from build123d import *

# Parameters (mm, degrees)
SKETCH1_W                   = 6.35
SKETCH1_H                   = 158.75
BOSS_EXTRUDE1_DEPTH         = 31.75
SKETCH2_R                   = 3.048
AXLE_HOLES_DEPTH            = 7.35
F_3_0MM_DOWEL_HOLE2_D       = 3
SKETCH4_W                   = 6.0325
SKETCH4_H                   = 6.638636364
CHEESING_CUT_DEPTH          = 5.334
FILLET1_R                   = 2.54
F_3_0MM_DOWEL_HOLE1_D       = 3
M3X0_5_TAPPED_HOLE3_D       = 3
M3X0_5_TAPPED_HOLE3_DEPTH   = 14.9999954
M3X0_5_TAPPED_HOLE3_TIP     = 0.901290929
HOLE_WIZARD_7903_AT_2_COUNT = 2
HOLE_WIZARD_7903_AT_2_PITCH = 12.636677574
F_3_0MM_DOWEL_HOLE4_D       = 3
CIRPATTERN1_COUNT           = 4


with BuildPart() as part:
    # Sketch1 → Boss-Extrude1 (new body)
    with BuildSketch(Plane(origin=(0, 0, 0), x_dir=(1, 0, 0), z_dir=(0, 1, 0))):
        with Locations((-3.175, -79.375)):
            Rectangle(SKETCH1_W, SKETCH1_H)
    extrude(amount=BOSS_EXTRUDE1_DEPTH)

    # Sketch2 → axle holes (cut, through all)
    with BuildSketch(Plane(origin=(0, 0, 0), x_dir=(0, 0, -1), z_dir=(1, 0, 0))):
        with Locations((-23.8125, 15.875)):
            Circle(SKETCH2_R)
        with Locations((-87.3125, 15.875)):
            Circle(SKETCH2_R)
        with Locations((-149.86, 15.875)):
            Circle(SKETCH2_R)
    extrude(amount=-AXLE_HOLES_DEPTH, mode=Mode.SUBTRACT)

    # Ø3.0mm Dowel Hole2 (through all)
    with Locations(Plane(origin=(0, 0, 0), x_dir=(0, 0, -1), z_dir=(1, 0, 0))):
        with Locations((-114.3, 3.175), (-95.25, 3.175)):
            f_3_0mm_dowel_hole2 = Hole(F_3_0MM_DOWEL_HOLE2_D / 2)

    # Sketch4 → cheesing cut (cut)
    with BuildSketch(Plane(origin=(0, 0, 0), x_dir=(0, 0, -1), z_dir=(1, 0, 0))):
        Polygon((-125.857199693, 15.875), (-142.24, 22.299627571), (-142.24, 9.450372429), align=None)
        Polygon((-101.568449693, 25.4), (-134.334050307, 25.4), (-117.95125, 18.975372429), align=None)
        Polygon((-93.6625, 22.299627571), (-110.045300307, 15.875), (-93.6625, 9.450372429), align=None)
        Polygon((-101.568449693, 6.35), (-117.95125, 12.774627571), (-134.334050307, 6.35), align=None)
        Polygon((-65.150024324, 15.875), (-80.9625, 22.285463112), (-80.9625, 9.464536888), align=None)
        Polygon((-41.655024324, 25.4), (-73.279975676, 25.4), (-57.4675, 18.989536888), align=None)
        Polygon((-33.9725, 22.285463112), (-49.784975676, 15.875), (-33.9725, 9.464536888), align=None)
        with Locations((-10.63625, 9.669318182)):
            Rectangle(SKETCH4_W, SKETCH4_H)
        with Locations((-10.63625, 22.080681818)):
            Rectangle(SKETCH4_W, SKETCH4_H)
    extrude(amount=-CHEESING_CUT_DEPTH, mode=Mode.SUBTRACT)

    # Fillet1
    fillet1_edges = [part.edges().sort_by_distance(p)[0] for p in [
        (-2.667, 22.285463112, 80.9625),
        (-2.667, 15.875, 65.150024324),
        (-2.667, 9.464536888, 80.9625),
        (-2.667, 12.774627571, 117.95125),
        (-2.667, 6.35, 101.568449693),
        (-2.667, 6.35, 134.334050307),
        (-2.667, 25.4, 134.334050307),
        (-2.667, 25.4, 101.568449693),
        (-2.667, 18.975372429, 117.95125),
        (-2.667, 22.299627571, 93.6625),
        (-2.667, 9.450372429, 93.6625),
        (-2.667, 15.875, 110.045300307),
        (-2.667, 15.875, 49.784975676),
        (-2.667, 22.285463112, 33.9725),
        (-2.667, 9.464536888, 33.9725),
        (-2.667, 25.4, 73.279975676),
        (-2.667, 25.4, 41.655024324),
        (-2.667, 18.989536888, 57.4675),
        (-2.667, 12.988636364, 13.6525),
        (-2.667, 12.988636364, 7.62),
        (-2.667, 6.35, 7.62),
        (-2.667, 6.35, 13.6525),
        (-2.667, 18.761363636, 13.6525),
        (-2.667, 25.4, 13.6525),
        (-2.667, 25.4, 7.62),
        (-2.667, 18.761363636, 7.62),
        (-2.667, 15.875, 125.857199693),
        (-2.667, 9.450372429, 142.24),
        (-2.667, 22.299627571, 142.24),
    ]]
    fillet(fillet1_edges, radius=FILLET1_R)

    # Mirror1: Ø3.0mm Dowel Hole2 across plane
    add(f_3_0mm_dowel_hole2.mirror(Plane.ZX.offset(15.875)), mode=Mode.SUBTRACT)

    # Ø3.0mm Dowel Hole1 (through all)
    with Locations(Plane(origin=(0, 0, 0), x_dir=(0, 0, -1), z_dir=(1, 0, 0))):
        with Locations((-69.685396292, 6), (-62.351396292, 6)):
            Hole(F_3_0MM_DOWEL_HOLE1_D / 2)

    # M3x0.5 Tapped Hole3
    with Locations(Plane(origin=(101.342838782, 5.251462055, -6.35), x_dir=(-1, 0, 0), z_dir=(0, 0, -1))):
        with Locations((104.517838782, 20.148537945), (104.517838782, 1.098537945)):
            Hole(M3X0_5_TAPPED_HOLE3_D / 2, depth=M3X0_5_TAPPED_HOLE3_DEPTH)
            with Locations((0, 0, -(M3X0_5_TAPPED_HOLE3_DEPTH + M3X0_5_TAPPED_HOLE3_TIP / 2))):  # 118° drill point
                Cone(0, M3X0_5_TAPPED_HOLE3_D / 2, M3X0_5_TAPPED_HOLE3_TIP, mode=Mode.SUBTRACT)

    # Sketch18 → Hole Wizard 7903 (revolve, cut)
    with BuildSketch(Plane(origin=(-3.236678341, -2.577911324, 139.812714896), x_dir=(0, -0.001998321, -0.999998003), z_dir=(1, 0, 0))):
        Polygon((0, 0), (0, 8.521290929), (1.5, 7.62), (1.5, 0), align=None)
    hole_wizard_7903 = revolve(axis=Axis((-3.236678341, -8.927898646, 139.825404238), (0, 0.999998003, -0.001998321)), mode=Mode.SUBTRACT)

    # Hole Wizard 7903 at 2: Hole Wizard 7903 ×2
    with Locations(*[Vector(0, 0.001998321, 0.999998003) * (i * HOLE_WIZARD_7903_AT_2_PITCH) for i in range(1, HOLE_WIZARD_7903_AT_2_COUNT)]):
        add(hole_wizard_7903, mode=Mode.SUBTRACT)

    # Mirror2: Hole Wizard 7903 across plane
    add(hole_wizard_7903.mirror(Plane.ZX.offset(15.875)), mode=Mode.SUBTRACT)

    # Mirror2 copy 1 sketch → Mirror2 copy 1 (revolve, cut)
    with BuildSketch(Plane(origin=(-3.236678341, 34.30265918, 152.449367239), x_dir=(0, 0.001998321, -0.999998003), z_dir=(1, 0, 0))):
        Polygon((0, 0), (0, -8.521290929), (1.5, -7.62), (1.5, 0), align=None)
    revolve(axis=Axis((-3.236678341, 40.652646501, 152.462056581), (0, 0.999998003, 0.001998321)), mode=Mode.SUBTRACT)

    # Ø3.0mm Dowel Hole4 (through all)
    with Locations(Plane(origin=(0, 0, 0), x_dir=(0, 0, -1), z_dir=(1, 0, 0))):
        with Locations((-30.1625, 22.225)):
            f_3_0mm_dowel_hole4 = Hole(F_3_0MM_DOWEL_HOLE4_D / 2)

    # CirPattern1: Ø3.0mm Dowel Hole4 ×4 about axis
    cirpattern1_axis = Axis((0, 15.875, 23.8125), (1, 0, 0))
    for i in range(1, CIRPATTERN1_COUNT):
        add(f_3_0mm_dowel_hole4.rotate(cirpattern1_axis, i * 360 / CIRPATTERN1_COUNT), mode=Mode.SUBTRACT)


solid = part.part
Input: part model. Units: mm. Frame: model coordinates. A direction names the side the tool comes from. Round coordinates to 2 decimals unless told otherwise and drop trailing zeros. Order: outer loops, then holes, each group sorted by start corner. A loop starts at its lowest first (then second) coordinate and runs counter-clockwise, first axis right, second up. Notation, with made-up numbers: (43, 87.5) - (91, 87.5) arc R23 cw to (91, 106.5) - close; hole circle Ø8 at (31.25, 46.5). An arc over 180 degrees is marked (long way). Answer as a JSON object with one key per item and string values. Group by question number.
(1) Pin query (flat end, axial travel): P1, Ø1.6, axis at x = -2, y = 16, coming from the -Z side; P2, Ø2.5, axis at y = 6, z = 62.35, coming from the -X side; P3, Ø3, axis at y = 18.5, z = 137, coming from the +X side. Return the tip coordinate at first contact, or that it passes through.
(2) Cut plane C-C (z = 149). Return loops of the section in (x, y).
(3) Reachability of faces 1 (the face through (-3.131, 16.009, 90.358)), 2 (the face through (-2.7, 23.3, 112.5)) from +Z, -Z, +X, -X, +Y, -Y: full face, straight path, thin tool, end or side. Return the list, or none.
(4) Draft query along Z for faces 3 (the face through (-3, 31.75, 78)), 4 (the face through (-3, 25.4, 57)). Return one class per face: released by +Z, released by -Z, zero draft, split by the parting line, or undercut.
(5) Cut plane B-B (z = 22.5). Return loops of the section in (x, y), then the cut area to 3 significant figures.
(6) Material intervals for probe 1 along Z at (x, y) = (-5.75, 9.5); probe 2 along Z at (x, y) = (-3, 28.5); probe 3 along Y at (x, z) = (-2, 95.25) (3 decimals), sorted ascending. Write a range as from..to.
(7) Cut plane A-A (z = 95.25). Return loops of the section in (x, y) (3 decimals).
Here are the results:
{
 "1": {"P1": "stops at z = 0", "P2": "passes through", "P3": "stops at x = -5.33"},
 "2": {"outline": "(-6.35, 0) - (0, 0) - (0, 12.95) - (-6.35, 12.95) - close; (-6.35, 18.8) - (0, 18.8) - (0, 31.75) - (-6.35, 31.75) - close"},
 "3": {"face 1": "+X, -X", "face 2": "+X"},
 "4": {"face 3": "zero draft", "face 4": "undercut"},
 "5": {"outline": "(-6.35, 0) - (0, 0) - (0, 13.12) - (-6.35, 13.12) - close; (-6.35, 18.63) - (0, 18.63) - (0, 31.75) - (-6.35, 31.75) - close", "area": "167 mm^2"},
 "6": {"probe 1": "z = 0..15.96, 18.96..28.66, 31.66..158.75", "probe 2": "z = 0..93.75, 96.75..112.8, 115.8..138.32, 141.28..150.96, 153.92..158.75", "probe 3": "y = 0..1.675, 4.675..10.82, 20.93..27.075, 30.075..31.75"},
 "7": {"outline": "(-6.35, 0) - (0, 0) - (0, 1.675) - (-6.35, 1.675) - close; (-6.35, 4.675) - (0, 4.675) - (0, 10.82) - (-5.334, 10.82) - (-5.334, 20.93) - (0, 20.93) - (0, 27.075) - (-6.35, 27.075) - close; (-6.35, 30.075) - (0, 30.075) - (0, 31.75) - (-6.35, 31.75) - close"}
}
